Source: CAD feature listing. Evaluate the final solid. Frame: model axes, mm. A direction names the side the tool comes from. Round coordinates to 2 decimals unless told otherwise and drop trailing zeros. Loops run counter-clockwise (first coordinate to the right, second up) from the corner with the lowest first, then second, coordinate; pieces in that order, holes last. Notation, with made-up numbers: (52.5, 53.5) -> (101.5, 53.5) arc R22 cw to (101.5, 77.5) -> close; hole circle Ø6 at (34.25, 70). An arc over 180 degrees is marked (long way). Put each result on its own line as item: value. Start each with the question number.
1. Set-up query: faces 1 (the flat face through (89, -2.4, 84)), 2 (the flat face through (0, 25, 84)), 3 (the flat face through (90, 1, 168)), 4 (the flat face through (90, 1, 2)). Return all of +Z, -Z, +X, -X, +Y, -Y with unobstructed straight access to the full face (end or side cutting, diameter ignored); none if empty.
2. Contact query for flat-ended pins moving along their axis: pin 1 (4 mm diameter, centred on x = 178, y = 4, fed in from -Z); pin 2 (1.6 mm diameter, centred on x = 65, z = 1, fed in from +Y); pin 3 (0.6 mm diameter, centred on x = 95.5, y = 1, fed in from +Z). Output: stop coordinate, or through.
3. Draft query along Z for faces 5 (the flat face through (182.8, 25, 84)), 6 (the flat face through (90, -2, 0)), 7 (the flat face through (4, 4, 7)). Return one class per face: pulls with the +Z half, pulls with the -Z half, needs draft (parallel to the pull), parting line crosses it, or undercut.
4. Cut plane C-C (x = 159). Return the cut outline in (y, z), then the cut area to 3 significant figures.
5. Material intervals for L1, parallel to X at y = 23, z = 59; L2, parallel to X at y = 2, z = 8; L3, parallel to Y at x = 46, z = 153.5, sorted ascending.
6. Cut plane A-A (y = 12.5). Return the cut outline in (x, z), then the cut area to 3 significant figures.
```python
from build123d import *

# Parameters (mm, degrees)
EXTRUDE_1_DEPTH = 170
EXTRUDE_START   = 2
SKETCH_1_3_R    = 1
EXTRUDE_2_DEPTH = 10
EXTRUDE_3_DEPTH = 2
FILLET_1_R      = 1
EXTRUDE_START_2 = 158
SKETCH_1_5_R    = 1
EXTRUDE_4_DEPTH = 10
EXTRUDE_START_3 = 166
EXTRUDE_5_DEPTH = 2
FILLET_2_R      = 1
SKETCH_2_W      = 1.2
SKETCH_2_H      = 170
EXTRUDE_6_DEPTH = 3
CHAMFER_1_SIZE2 = 3
CHAMFER_1_SIZE  = 0.262465991
CHAMFER_2_SIZE2 = 0.262465991
CHAMFER_2_SIZE  = 3
FILLET_3_R      = 1


with BuildPart() as part:
    # Эскиз1 → Бобышка-Вытянуть1 (new body)
    with BuildSketch(Plane.XY):
        Polygon((0, 49.2), (-2.4, 49.2), (-2.4, -2.4), (182.8, -2.4), (182.8, 49.2), (180.4, 49.2), (180.4, 0), (0, 0), align=None)
    extrude(amount=EXTRUDE_1_DEPTH)

    # Эскиз1<3> → Бобышка-Вытянуть2 (add)
    # profile 1 of 2: a face of its own
    with BuildSketch(Plane.XY.offset(EXTRUDE_START)):
        Polygon((2, 6), (0, 8), (0, 0), (8, 0), (6, 2), align=None)
        with Locations((2.7, 2.7)):
            Circle(SKETCH_1_3_R, mode=Mode.SUBTRACT)
    # profile 2 of 2: a face of its own
    with BuildSketch(Plane.XY.offset(EXTRUDE_START)):
        Polygon((174.4, 2), (172.4, 0), (180.4, 0), (180.4, 8), (178.4, 6), align=None)
        with Locations((177.7, 2.7)):
            Circle(SKETCH_1_3_R, mode=Mode.SUBTRACT)
    extrude(amount=EXTRUDE_2_DEPTH)

    # Эскиз1<4> → Бобышка-Вытянуть3 (add)
    with BuildSketch(Plane.XY.offset(EXTRUDE_START)):
        Polygon((178.4, 49.2), (178.4, 6), (180.4, 8), (180.4, 49.2), align=None)
        Polygon((6, 2), (8, 0), (172.4, 0), (174.4, 2), align=None)
        Polygon((2, 49.2), (0, 49.2), (0, 8), (2, 6), align=None)
    extrude(amount=EXTRUDE_3_DEPTH)

    # Скругление1
    fillet_1_edges = [part.edges().sort_by_distance(p)[0] for p in [
        (182.8, -2.4, 85),
        (-2.4, -2.4, 85),
        (0, 0, 1),
        (180.4, 0, 1),
    ]]
    fillet(fillet_1_edges, radius=FILLET_1_R)

    # Эскиз1<5> → Бобышка-Вытянуть4 (add)
    # profile 1 of 2: a face of its own
    with BuildSketch(Plane.XY.offset(EXTRUDE_START_2)):
        Polygon((174.4, 2), (172.4, 0), (180.4, 0), (180.4, 8), (178.4, 6), align=None)
        with Locations((177.7, 2.7)):
            Circle(SKETCH_1_5_R, mode=Mode.SUBTRACT)
    # profile 2 of 2: a face of its own
    with BuildSketch(Plane.XY.offset(EXTRUDE_START_2)):
        Polygon((2, 6), (0, 8), (0, 0), (8, 0), (6, 2), align=None)
        with Locations((2.7, 2.7)):
            Circle(SKETCH_1_5_R, mode=Mode.SUBTRACT)
    extrude(amount=EXTRUDE_4_DEPTH)

    # Эскиз1<6> → Бобышка-Вытянуть5 (add)
    with BuildSketch(Plane.XY.offset(EXTRUDE_START_3)):
        Polygon((178.4, 49.2), (178.4, 6), (180.4, 8), (180.4, 49.2), align=None)
        Polygon((6, 2), (8, 0), (172.4, 0), (174.4, 2), align=None)
        Polygon((2, 49.2), (0, 49.2), (0, 8), (2, 6), align=None)
    extrude(amount=EXTRUDE_5_DEPTH)

    # Скругление2
    fillet_2_edges = [part.edges().sort_by_distance(p)[0] for p in [
        (180.4, 0, 85),
        (0, 0, 85),
    ]]
    fillet(fillet_2_edges, radius=FILLET_2_R)

    # Эскиз2 → Бобышка-Вытянуть6 (add)
    with BuildSketch(Plane(origin=(0, 49.2, 0), x_dir=(1, 0, 0), z_dir=(0, 1, 0))):
        with Locations((-1.8, -85)):
            Rectangle(SKETCH_2_W, SKETCH_2_H)
        with Locations((182.2, -85)):
            Rectangle(SKETCH_2_W, SKETCH_2_H)
    extrude(amount=EXTRUDE_6_DEPTH)

    # Фаска1
    chamfer_1_edges = [part.edges().sort_by_distance(p)[0] for p in [
        (-1.2, 52.2, 85),
    ]]
    chamfer_1_side = [part.faces().sort_by_distance(p)[0] for p in [
        (-1.20524932, 52.2, 85),
    ]]
    chamfer(chamfer_1_edges, length=CHAMFER_1_SIZE - 0.0001, length2=CHAMFER_1_SIZE2 - 0.0001, reference=chamfer_1_side[0])  # a hair under: the kernel refuses the full size

    # Фаска2
    chamfer_2_edges = [part.edges().sort_by_distance(p)[0] for p in [
        (181.6, 52.2, 85),
    ]]
    chamfer_2_side = [part.faces().sort_by_distance(p)[0] for p in [
        (181.6, 52.19475068, 85),
    ]]
    chamfer(chamfer_2_edges, length=CHAMFER_2_SIZE - 0.0001, length2=CHAMFER_2_SIZE2 - 0.0001, reference=chamfer_2_side[0])  # a hair under: the kernel refuses the full size

    # Скругление3
    fillet_3_edges = [part.edges().sort_by_distance(p)[0] for p in [
        (0, 0, 169),
        (180.4, 0, 169),
    ]]
    fillet(fillet_3_edges, radius=FILLET_3_R)


solid = part.part
```
Solution:
1. face 1: +Z, -Z, +X, -X, -Y
1. face 2: +Y
1. face 3: +Z, +Y
1. face 4: -Z, +Y
2. pin 1: stops at z = 2
2. pin 2: stops at y = 0
2. pin 3: stops at z = 168
3. face 5: needs draft
3. face 6: pulls with the -Z half
3. face 7: undercut
4. outline: (-2.4, 0) -> (0, 0) -> (0, 2) -> (2, 2) -> (2, 4) -> (0, 4) -> (0, 166) -> (2, 166) -> (2, 168) -> (0, 168) -> (0, 170) -> (-2.4, 170) -> close
4. area: 416 mm^2
5. L1: x = -2.4 to 0, 180.4 to 182.8
5. L2: x = -2.4 to 1.99, 3.41 to 6, 174.4 to 176.99, 178.41 to 182.8
5. L3: y = -2.4 to 0
6. outline: (-2.4, 0) -> (0, 0) -> (0, 2) -> (2, 2) -> (2, 4) -> (0, 4) -> (0, 166) -> (2, 166) -> (2, 168) -> (0, 168) -> (0, 170) -> (-2.4, 170) -> close; (178.4, 2) -> (180.4, 2) -> (180.4, 0) -> (182.8, 0) -> (182.8, 170) -> (180.4, 170) -> (180.4, 168) -> (178.4, 168) -> (178.4, 166) -> (180.4, 166) -> (180.4, 4) -> (178.4, 4) -> close
6. area: 832 mm^2
